Can you work these out from the model? Positions are in its coordinate system, mm. A direction names the side the tool comes from. Give positions to 0.01 mm unless a question says otherwise; leave off trailing zeros. Loops run counter-clockwise (first coordinate to the right, second up) from the corner with the lowest first, then second, coordinate; pieces in that order, holes last. Notation, with made-up numbers: (85, -39) - (120, -39) arc R33 cw to (120, -6) - close; hole circle Ø6 at (58, -38). An arc over 180 degrees is marked (long way). Use a Markdown table: item, result. Add a question column.
```python
from build123d import *

# Parameters (mm, degrees)
SKETCH1_W                  = 74.5
SKETCH1_H                  = 42.8
BOSS_EXTRUDE1_DEPTH        = 1.6002
SKETCH2_W                  = 60.3
SKETCH2_H                  = 42.8
BOSS_EXTRUDE2_DEPTH        = 4.2
F_3_2_3_2_DIAMETER_HOLE1_D = 3.2
FILLET1_R                  = 3
SKETCH6_W                  = 8
SKETCH6_H                  = 15
BOSS_EXTRUDE3_DEPTH        = 6.25
SKETCH7_W                  = 5.7
SKETCH7_H                  = 12.3
BOSS_EXTRUDE4_DEPTH        = 3.5
SKETCH8_W                  = 14.9
SKETCH8_H                  = 14.75
BOSS_EXTRUDE5_DEPTH        = 2.15
SKETCH9_W                  = 11.03
SKETCH9_H                  = 1.1
BOSS_EXTRUDE6_DEPTH        = 2.5


with BuildPart() as part:
    # Sketch1 → Boss-Extrude1 (new body)
    with BuildSketch(Plane.XY):
        Rectangle(SKETCH1_W, SKETCH1_H)
    extrude(amount=-BOSS_EXTRUDE1_DEPTH)

    # Sketch2 → Boss-Extrude2 (add)
    with BuildSketch(Plane.XY):
        with Locations((-0.04, 0)):
            Rectangle(SKETCH2_W, SKETCH2_H)
    extrude(amount=BOSS_EXTRUDE2_DEPTH)

    # Ø3.2 (3.2) Diameter Hole1 (through all)
    with Locations(Plane.XY):
        with Locations((-34.16, 18.245), (34.16, -18.245), (34.16, 18.245), (-34.16, -18.245)):
            Hole(F_3_2_3_2_DIAMETER_HOLE1_D / 2)

    # Fillet1
    fillet1_edges = [part.edges().sort_by_distance(p)[0] for p in [
        (37.25, 21.4, -0.8001),
        (37.25, -21.4, -0.8001),
        (-37.25, -21.4, -0.8001),
        (-37.25, 21.4, -0.8001),
    ]]
    fillet(fillet1_edges, radius=FILLET1_R)

    # Sketch6 → Boss-Extrude3 (add)
    with BuildSketch(Plane(origin=(0, 0, -1.6002), x_dir=(-1, 0, 0), z_dir=(0, 0, -1))):
        with Locations((33.25, 0)):
            Rectangle(SKETCH6_W, SKETCH6_H)
    extrude(amount=BOSS_EXTRUDE3_DEPTH)

    # Sketch7 → Boss-Extrude4 (add)
    with BuildSketch(Plane.ZY.offset(37.25)):
        with Locations((-4.9902, 0)):
            Rectangle(SKETCH7_W, SKETCH7_H)
    extrude(amount=BOSS_EXTRUDE4_DEPTH)

    # Sketch8 → Boss-Extrude5 (add)
    with BuildSketch(Plane(origin=(0, 0, -1.6002), x_dir=(-1, 0, 0), z_dir=(0, 0, -1))):
        with Locations((16, -14.025)):
            Rectangle(SKETCH8_W, SKETCH8_H)
    extrude(amount=BOSS_EXTRUDE5_DEPTH)

    # Sketch9 → Boss-Extrude6 (add)
    with BuildSketch(Plane.XZ.offset(21.4)):
        with Locations((-14.835, -3.1902)):
            Rectangle(SKETCH9_W, SKETCH9_H)
    extrude(amount=BOSS_EXTRUDE6_DEPTH)


solid = part.part
```
1. Please list where these lines run through material, in increasing order: line 1 along Y through (x, z) = (-34.16, -1.05) (3 decimals); line 2 along Z through (x, y) = (-28, -8); line 3 along Y through (x, z) = (-22.5, 3.5). Write a range as [from, to].
2. Will these pins go through, and if not, where does the flat tip stop? P1, Ø4, axis at x = 34.16, y = -18.245, coming from the -Z side; P2, Ø1.8, axis at x = -39, y = 2, coming from the -Z side; P3, Ø1.5, axis at y = 1.5, z = 1, coming from the +X side.
3. Suppose I cut it at B-B (z = -5.5). List the corners of the cut face in (x, y) for me.
4. If we mould it in two halves opening along X, with no side actions, what happens to faces 5 (the face through (-32.56, 18.32, -0.81)), 6 (the face through (-33, 0, -7.85)), 7 (the face through (37.25, 0, -1))? For each: released by +X, released by -X, zero draft, split by the parting line, or undercut.
5. On a 3-axis mill with a long thin cutter (end or side, diameter ignored), from which of +Z, -Z, +X, -X, +Y, -Y can I reach the whole of each face in a straight line? I mean faces 1 (the face through (30.11, 0, 2)), 2 (the face through (-33, -7.5, -5)), 3 (the face through (-30.19, 0, 2)), 4 (the face through (-15, -23, -2.64)). Say none if no direction works.
6. Suppose I cut it at A-A (x = -31). List the corners of the cut face in (y, z) for me, and give its area (3 significant figures).
Results below:
| question | item | result |
|---|---|---|
| 1 | line 1 | [-21.4, -19.845], [-16.645, 16.645], [19.845, 21.4] |
| 1 | line 2 | [-1.6, 4.2] |
| 1 | line 3 | [-21.4, 21.4] |
| 2 | P1 | z = -1.6 |
| 2 | P2 | z = -7.84 |
| 2 | P3 | x = 30.11 |
| 3 | outline | (-40.75, -6.15) - (-37.25, -6.15) - (-37.25, -7.5) - (-29.25, -7.5) - (-29.25, 7.5) - (-37.25, 7.5) - (-37.25, 6.15) - (-40.75, 6.15) - close |
| 4 | face 5 | undercut |
| 4 | face 6 | zero draft |
| 4 | face 7 | released by +X |
| 5 | face 1 | +Z, +X, +Y, -Y |
| 5 | face 2 | -Z, -X, -Y |
| 5 | face 3 | +Z, -X, +Y, -Y |
| 5 | face 4 | +Z, +X, -X, -Y |
| 6 | outline | (-21.4, -1.6) - (-7.5, -1.6) - (-7.5, -7.85) - (7.5, -7.85) - (7.5, -1.6) - (21.4, -1.6) - (21.4, 0) - (-21.4, 0) - close |
| 6 | area | 162 mm² |
